from build123d import *

# Parameters (mm, degrees)
SKETCH_W        = 95
SKETCH_H        = 27
PAD_DEPTH       = 2
SKETCH001_R     = 1.3
POCKET_DEPTH    = 2
FILLET_R        = 3
SKETCH002_W     = 9.2
SKETCH002_H     = 11.4
POCKET001_DEPTH = 2
SKETCH004_W     = 43.25
SKETCH004_H     = 11.5
POCKET002_DEPTH = 2
POCKET003_DEPTH = 2


with BuildPart() as part:
    # Sketch → Pad (new body)
    with BuildSketch(Plane.XY):
        Rectangle(SKETCH_W, SKETCH_H)
    extrude(amount=PAD_DEPTH)

    # Sketch001 (on Face6 of Pad) → Pocket (cut)
    with BuildSketch(Plane.XY.offset(2)):
        with Locations((-44.5, 10.5)):
            Circle(SKETCH001_R)
        with Locations((44.5, 10.5)):
            Circle(SKETCH001_R)
        with Locations((44.5, -10.5)):
            Circle(SKETCH001_R)
        with Locations((-44.5, -10.5)):
            Circle(SKETCH001_R)
    extrude(amount=-POCKET_DEPTH, mode=Mode.SUBTRACT)

    # Fillet
    fillet_edges = [part.edges().sort_by_distance(p)[0] for p in [
        (-47.5, -13.5, 1),
        (47.5, -13.5, 1),
        (47.5, 13.5, 1),
        (-47.5, 13.5, 1),
    ]]
    fillet(fillet_edges, radius=FILLET_R)

    # Sketch002 (on Face5 of Fillet) → Pocket001 (cut)
    with BuildSketch(Plane.XY.offset(2)):
        with Locations((31.3, 1.1)):
            Rectangle(SKETCH002_W, SKETCH002_H)
    extrude(amount=-POCKET001_DEPTH, mode=Mode.SUBTRACT)

    # Sketch004 (on Face5 of Pocket001) → Pocket002 (cut)
    with BuildSketch(Plane.XY.offset(2)):
        with Locations((-18.875, 1.15)):
            Rectangle(SKETCH004_W, SKETCH004_H)
    extrude(amount=-POCKET002_DEPTH, mode=Mode.SUBTRACT)

    # Sketch005 (on Face5 of Pocket002) → Pocket003 (cut)
    with BuildSketch(Plane.XY.offset(2)):
        Polygon((16.15, 1.7), (16.15, -6.1), (3.4, -6.1), (3.4, 1.7), (6.4, 1.7), (6.4, 2.5), (13.15, 2.5), (13.15, 1.7), align=None)
    extrude(amount=-POCKET003_DEPTH, mode=Mode.SUBTRACT)


solid = part.part
The listing builds one solid part. Answer for the finished solid, in the listing's coordinates (mm). A direction names the side the tool comes from. Round coordinates to 2 decimals unless told otherwise and drop trailing zeros. Loops run counter-clockwise (first coordinate to the right, second up) from the corner with the lowest first, then second, coordinate; pieces in that order, holes last. Notation, with made-up numbers: M 16,-3 L 67,-3 A32 ccw 67,33 Z; hole C 36.25,-21 d5. An arc over 180 degrees is marked long. Return JSON: item names as keys, results as strings.
Q1. This flat-tipped pin is pushed along its axis until it touches: pin 1 Ø10 at (x, y) = (-31, 1) entering from -Z. Where does it stop, or does it pass through?
Results list:
{"pin 1": "passes through"}
Q2. The mould has two halves that part along Y. Classify faces 1 (the face through (-46.64, 12.6, 1.01)), 2 (the face through (-1, -6, 0)), 3 (the face through (10, -6.1, 1)): released by +Y, released by -Y, zero draft, split by the parting line, or undercut.
Results list:
{"face 1": "released by +Y", "face 2": "zero draft", "face 3": "undercut"}
Q3. Find section B-B, the plane y = -3. Determine the outline of the cut face in (x, z), plus the area to 3 significant figures.
Results list:
{"outline": "M -47.5,0 L -40.5,0 L -40.5,2 L -47.5,2 Z; M 2.75,0 L 3.4,0 L 3.4,2 L 2.75,2 Z; M 16.15,0 L 26.7,0 L 26.7,2 L 16.15,2 Z; M 35.9,0 L 47.5,0 L 47.5,2 L 35.9,2 Z", "area": "59.6 mm2"}
Q4. Find section C-C, the plane x = 30. Determine the outline of the cut face in (y, z).
Results list:
{"outline": "M -13.5,0 L -4.6,0 L -4.6,2 L -13.5,2 Z; M 6.8,0 L 13.5,0 L 13.5,2 L 6.8,2 Z"}
Q5. Find section A-A, the plane x = -24. Determine the outline of the cut face in (y, z).
Results list:
{"outline": "M -13.5,0 L -4.6,0 L -4.6,2 L -13.5,2 Z; M 6.9,0 L 13.5,0 L 13.5,2 L 6.9,2 Z"}
Q6. Which of the six approach directions +Z, -Z, +X, -X, +Y, -Y give full straight-line access (tool end or side, diameter ignored) to faces 4 (the face through (-1, 13.5, 1)), 5 (the face through (26.7, 1, 1))?
Results list:
{"face 4": "+Z, -Z, +X, -X, +Y", "face 5": "+Z, -Z"}
Q7. Find the intervals of material crossed by line 1 along X through (y, z) = (-3, 0.3); line 2 along Y through (x, z) = (44.5, 1.05); line 3 along Y through (x, z) = (-17.5, 0.95), in increasing order. Write a range as from..to.
Results list:
{"line 1": "x = -47.5..-40.5, 2.75..3.4, 16.15..26.7, 35.9..47.5", "line 2": "y = -13.5..-11.8, -9.2..9.2, 11.8..13.5", "line 3": "y = -13.5..-4.6, 6.9..13.5"}
